```python
from build123d import *

# Parameters (mm, degrees)
SKETCH5_R           = 1.5
BOSS_EXTRUDE2_DEPTH = 3
SKETCH6_R           = 1.5
BOSS_EXTRUDE3_DEPTH = 11


with BuildPart() as part:
    # Sketch5 → Boss-Extrude2 (new body)
    with BuildSketch(Plane(origin=(0, 0, 0), x_dir=(1, 0, 0), z_dir=(0, 1, 0))):
        with BuildLine():
            Line((-5.196152423, 22.5), (-29.5, 22.5))
            ThreePointArc((-29.5, 22.5), (-31.621320344, 21.621320344), (-32.5, 19.5))
            Line((-32.5, 19.5), (-32.5, -17.303847577))
            ThreePointArc((-32.5, -17.303847577), (-32.901923789, -18.803847577), (-34, -19.901923789))
            ThreePointArc((-34, -19.901923789), (-35.397777479, -23.276457135), (-32.5, -25.5))
            Line((-32.5, -25.5), (32.5, -25.5))
            ThreePointArc((32.5, -25.5), (34.621320344, -24.621320344), (35.5, -22.5))
            Line((35.5, -22.5), (35.5, 22.5))
            ThreePointArc((35.5, 22.5), (34.621320344, 24.621320344), (32.5, 25.5))
            Line((32.5, 25.5), (0, 25.5))
            ThreePointArc((0, 25.5), (-1.5, 25.098076211), (-2.598076211, 24))
            ThreePointArc((-2.598076211, 24), (-3.696152423, 22.901923789), (-5.196152423, 22.5))
        make_face()
        with Locations(Location((0, 22.5, 0), (0, 0, 270))):
            Circle(SKETCH5_R, mode=Mode.SUBTRACT)
        with Locations(Location((32.5, 22.5, 0), (0, 0, 270))):
            Circle(SKETCH5_R, mode=Mode.SUBTRACT)
        with Locations(Location((32.5, -22.5, 0), (0, 0, 270))):
            Circle(SKETCH5_R, mode=Mode.SUBTRACT)
        with Locations(Location((-32.5, -22.5, 0), (0, 0, 270))):
            Circle(SKETCH5_R, mode=Mode.SUBTRACT)
    extrude(amount=BOSS_EXTRUDE2_DEPTH)

    # Sketch6 → Boss-Extrude3 (add)
    with BuildSketch(Plane(origin=(0, 3, 0), x_dir=(1, 0, 0), z_dir=(0, 1, 0))):
        with BuildLine():
            Line((-32.5, 5.885087138), (-32.5, -17.303847577))
            ThreePointArc((-32.5, -17.303847577), (-32.901923789, -18.803847577), (-34, -19.901923789))
            ThreePointArc((-34, -19.901923789), (-34.621320344, -24.621320344), (-29.901923789, -24))
            ThreePointArc((-29.901923789, -24), (-28.803847577, -22.901923789), (-27.303847577, -22.5))
            Line((-27.303847577, -22.5), (27.303847577, -22.5))
            ThreePointArc((27.303847577, -22.5), (28.803847577, -22.901923789), (29.901923789, -24))
            ThreePointArc((29.901923789, -24), (34.621320344, -24.621320344), (34, -19.901923789))
            ThreePointArc((34, -19.901923789), (32.901923789, -18.803847577), (32.5, -17.303847577))
            Line((32.5, -17.303847577), (32.5, 17.303847577))
            ThreePointArc((32.5, 17.303847577), (32.901923789, 18.803847577), (34, 19.901923789))
            ThreePointArc((34, 19.901923789), (34.621320344, 24.621320344), (29.901923789, 24))
            ThreePointArc((29.901923789, 24), (28.803847577, 22.901923789), (27.303847577, 22.5))
            Line((27.303847577, 22.5), (5.196152423, 22.5))
            ThreePointArc((5.196152423, 22.5), (3.696152423, 22.901923789), (2.598076211, 24))
            ThreePointArc((2.598076211, 24), (0, 25.5), (-2.598076211, 24))
            ThreePointArc((-2.598076211, 24), (-3.696152423, 22.901923789), (-5.196152423, 22.5))
            Line((-5.196152423, 22.5), (-18.854157071, 22.5))
            ThreePointArc((-18.854157071, 22.5), (-19.561263852, 22.207106781), (-19.854157071, 21.5))
            Line((-19.854157071, 21.5), (-19.854157071, 21))
            ThreePointArc((-19.854157071, 21), (-19.561263852, 20.292893219), (-18.854157071, 20))
            Line((-18.854157071, 20), (28, 20))
            ThreePointArc((28, 20), (29.414213562, 19.414213562), (30, 18))
            Line((30, 18), (30, -18))
            ThreePointArc((30, -18), (29.414213562, -19.414213562), (28, -20))
            Line((28, -20), (-28, -20))
            ThreePointArc((-28, -20), (-29.414213562, -19.414213562), (-30, -18))
            Line((-30, -18), (-30, 5.885087138))
            ThreePointArc((-30, 5.885087138), (-30.292893219, 6.592193919), (-31, 6.885087138))
            Line((-31, 6.885087138), (-31.5, 6.885087138))
            ThreePointArc((-31.5, 6.885087138), (-32.207106781, 6.592193919), (-32.5, 5.885087138))
        make_face()
        with Locations(Location((0, 22.5, 0), (0, 0, 270))):
            Circle(SKETCH6_R, mode=Mode.SUBTRACT)
        with Locations(Location((32.5, 22.5, 0), (0, 0, 270))):
            Circle(SKETCH6_R, mode=Mode.SUBTRACT)
        with Locations(Location((32.5, -22.5, 0), (0, 0, 270))):
            Circle(SKETCH6_R, mode=Mode.SUBTRACT)
        with Locations(Location((-32.5, -22.5, 0), (0, 0, 270))):
            Circle(SKETCH6_R, mode=Mode.SUBTRACT)
    extrude(amount=BOSS_EXTRUDE3_DEPTH)


solid = part.part
```
Source: CAD feature listing. Evaluate the final solid. Frame: model axes, mm. A direction names the side the tool comes from. Coordinates: 2 decimals unless noted, no trailing zeros. Loops run counter-clockwise (first coordinate to the right, second up) from the corner with the lowest first, then second, coordinate; pieces in that order, holes last. Notation, with made-up numbers: M 41.5,50.25 L 95.5,50.25 A27 ccw 95.5,88.25 Z; hole C 60.5,57.25 d8. An arc over 180 degrees is marked long. Use a Markdown table: item, result. Add a question column.
Q1. Access query for faces 4 (the flat face through (0, 3, 24)), 5 (the cylindrical face through (-29.4, 8.42, 19.43)), 6 (the flat face through (30, 8, 0)), 7 (the flat face through (4, 8, -20)). Directions: +Z, -Z, +X, -X, +Y, -Y. A direction counts if a zero-diameter tool reaches every point of the face in a straight line with its end or side. Return the directions, or none.
Q2. First-contact query: pin 1 (5.5 mm diameter, centred on y = 6, z = 6.5, fed in from +X); pin 2 (6 mm diameter, centred on y = 3.5, z = -2, fed in from -X); pin 3 (0.6 mm diameter, centred on x = -31.5, y = 8, fed in from -Z). Flat tips, straight axial feed; report the tip coordinate or a pass-through.
Q3. Section query D-D, the plane x = 12.5. Return loops of the section in (y, z).
Q4. Section query B-B, the plane y = 7.75. State how many separate pieces and enclosed holes the cut face has, and give its area (3 significant figures).
Q5. Section query A-A, the plane z = 16. Return loops of the section in (x, y), and give its area (3 significant figures).
Q6. Section query C-C, the plane x = -10. Return loops of the section in (y, z), and give its area (3 significant figures).
Q7. Draft query along Z for faces 1 (the flat face through (32.5, 8, 0)), 2 (the flat face through (0, 1, 25.5)), 3 (the flat face through (16, 8, -22.5)). Return one class per face: pulls with the +Z half, pulls with the -Z half, needs draft (parallel to the pull), parting line crosses it, or undercut.
Q8. Material intervals for L1, parallel to Z at x = 15, y = 6.5; L2, parallel to X at y = 4, z = 10.5; L3, parallel to X at y = 5.5, z = 22, sorted ascending.
Result:
| question | item | result |
|---|---|---|
| 1 | face 4 | +Z, +Y |
| 1 | face 5 | -Z, +Y |
| 1 | face 6 | +Y |
| 1 | face 7 | -X, +Y |
| 2 | pin 1 | stops at x = 32.5 |
| 2 | pin 2 | stops at x = -32.5 |
| 2 | pin 3 | stops at z = -6.89 |
| 3 | outline | M 0,-25.5 L 3,-25.5 L 3,-22.5 L 14,-22.5 L 14,-20 L 3,-20 L 3,20 L 14,20 L 14,22.5 L 3,22.5 L 3,25.5 L 0,25.5 Z |
| 4 | separate pieces | 1 |
| 4 | enclosed holes | 4 |
| 4 | area | 518 mm2 |
| 5 | outline | M -32.5,0 L 35.5,0 L 35.5,3 L 32.5,3 L 32.5,14 L 30,14 L 30,3 L -30,3 L -30,14 L -32.5,14 Z |
| 5 | area | 259 mm2 |
| 6 | outline | M 0,-22.5 L 14,-22.5 L 14,-20 L 3,-20 L 3,20 L 14,20 L 14,22.5 L 3,22.5 L 3,25.5 L 0,25.5 Z |
| 6 | area | 199 mm2 |
| 7 | face 1 | undercut |
| 7 | face 2 | pulls with the +Z half |
| 7 | face 3 | pulls with the -Z half |
| 8 | L1 | z = -22.5 to -20, 20 to 22.5 |
| 8 | L2 | x = -32.5 to -30, 30 to 32.5 |
| 8 | L3 | x = -35.46 to -33.91, -31.09 to 31.09, 33.91 to 35.46 |
